Design review of the part shown in the three views and the two pictorial views. Dimensions are in mm from the part's minimum x, y and z. Round coordinates to 2 decimals unless told otherwise and drop trailing zeros. Write each loop counter-clockwise with the first axis right and the second up, starting at its lowest first coordinate (ties: lowest second). Pieces come first, ordered by that corner, then holes. Notation, with made-up numbers: (-27.75, -27) - (17.25, -27) arc R24 ccw to (17.25, 9) - close; hole circle Ø10 at (58, 49.25). An arc over 180 degrees is marked (long way). Use one line per item in the form item = value.
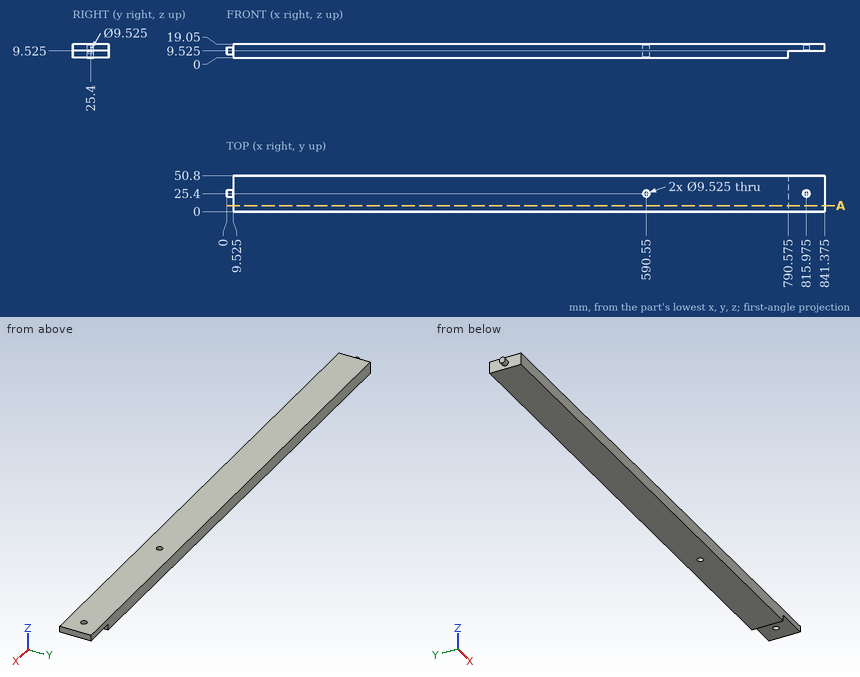
(1) To check wall thickness, follow L1, parallel to Y at x = 590.55, z = 5.75; L2, parallel to X at y = 37.5, z = 7.5 (3 decimals); L3, parallel to X at y = 46, z = 13.5 (3 decimals). State the ranges of each line that lie inside material, in increasing order.
Geometry results:
L1 = 0 to 20.64, 30.16 to 50.8
L2 = 9.525 to 790.575
L3 = 9.525 to 841.375
(2) Add section A-A on y = 8.5. Write out the cut boundary in (x, z) (3 decimals).
Geometry results:
outline = (9.525, 0) - (790.575, 0) - (790.575, 9.525) - (841.375, 9.525) - (841.375, 19.05) - (9.525, 19.05) - close
(3) Insertion check: P1, Ø4, axis at y = 16, z = 8.5, coming from the -X side (3 decimals); P2, Ø8, axis at y = 37, z = 4.5, coming from the +X side (3 decimals). Each pin has a flat end and moves straight along its axis. Give the tip position at first contact, or say it passes through.
Geometry results:
P1 = 9.525
P2 = 790.575
